Source: CAD feature listing. Evaluate the final solid. Frame: model axes, mm. A direction names the side the tool comes from. Give positions to 0.01 mm unless a question says otherwise; leave off trailing zeros. Order: outer loops, then holes, each group sorted by start corner. A loop starts at its lowest first (then second) coordinate and runs counter-clockwise, first axis right, second up. Notation, with made-up numbers: M 31,85.25 L 85,85.25 A12 ccw 85,108.25 Z; hole C 31.5,47 d1. An arc over 180 degrees is marked long. Answer in a Markdown table with one row per item. Add a question column.
(1) Mould query, pull axis X, two halves, no side actions, for faces 1 (the face through (3.45, -4.93, 0.74)), 2 (the face through (20, -23, 1.5)), 3 (the face through (40, -49, 2)). Classes: pulls with the +X half, pulls with the -X half, needs draft (parallel to the pull), parting line crosses it, or undercut.
(2) Material intervals for line 1 along Y through (x, z) = (5, 0.3); line 2 along Y through (x, z) = (35, 2); line 3 along Z through (x, y) = (13, -20.5), sorted ascending.
(3) Section query B-B, the plane z = 3.5. Return loops of the section in (x, y).
(4) Section query C-C, the plane y = -12. Return loops of the section in (x, z), plus the area to 3 significant figures.
(5) Set-up query: faces 4 (the face through (20, -46, 4)), 5 (the face through (36.478, -4.534, 0.74)). Return all of +Z, -Z, +X, -X, +Y, -Y with unobstructed straight access to the full face (end or side cutting, diameter ignored); none if empty.
(6) Pin query (flat end, axial travel): P1, Ø3.5, axis at x = 35, y = -35, coming from the +Z side; P2, Ø3, axis at x = 5, y = -35, coming from the +Z side; P3, Ø1.5, axis at x = 16.5, z = 5, coming from the +Y side. Return the tip coordinate at first contact, or that it passes through.
(7) Section query A-A, the plane y = -35. Return loops of the section in (x, z), plus the area to 3 significant figures.
from build123d import *

# Parameters (mm, degrees)
SKETCH_1_W          = 40
SKETCH_1_H          = 70
SKETCH_1_R          = 1.55
EXTRUDE_1_DEPTH     = 1.5
SKETCH_2_W          = 40
SKETCH_2_H          = 24
EXTRUDE_2_DEPTH     = 5
SKETCH_3_R          = 1.55
CUT_EXTRUDE_1_DEPTH = 25
FILLET_1_R          = 5


with BuildPart() as part:
    # 草图1 → 凸台-拉伸1 (new body)
    with BuildSketch(Plane.XY):
        with Locations((20, -35)):
            Rectangle(SKETCH_1_W, SKETCH_1_H)
        with Locations((5, -5)):
            Circle(SKETCH_1_R, mode=Mode.SUBTRACT)
        with Locations((35, -5)):
            Circle(SKETCH_1_R, mode=Mode.SUBTRACT)
        with Locations((5, -35)):
            Circle(SKETCH_1_R, mode=Mode.SUBTRACT)
        with Locations((35, -35)):
            Circle(SKETCH_1_R, mode=Mode.SUBTRACT)
        with Locations((5, -65)):
            Circle(SKETCH_1_R, mode=Mode.SUBTRACT)
        with Locations((35, -65)):
            Circle(SKETCH_1_R, mode=Mode.SUBTRACT)
    extrude(amount=EXTRUDE_1_DEPTH)

    # 草图2 → 凸台-拉伸2 (add)
    with BuildSketch(Plane.XY.offset(1.5)):
        with Locations((20, -58)):
            Rectangle(SKETCH_2_W, SKETCH_2_H)
    extrude(amount=EXTRUDE_2_DEPTH)

    # 草图3 → 切除-拉伸1 (cut)
    with BuildSketch(Plane(origin=(0, 0, 1.5), x_dir=(-1, 0, 0), z_dir=(0, 0, -1))):
        with Locations(Location((-35, -65, 0), (0, 0, 180))):
            Circle(SKETCH_3_R)
        with Locations(Location((-5, -65, 0), (0, 0, 180))):
            Circle(SKETCH_3_R)
    extrude(amount=-CUT_EXTRUDE_1_DEPTH, mode=Mode.SUBTRACT)

    # 圆角1
    fillet_1_edges = [part.edges().sort_by_distance(p)[0] for p in [
        (0, 0, 0.75),
        (40, 0, 0.75),
        (40, -70, 3.25),
        (0, -70, 3.25),
    ]]
    fillet(fillet_1_edges, radius=FILLET_1_R)


solid = part.part
Values follow:
| question | item | result |
|---|---|---|
| 1 | face 1 | undercut |
| 1 | face 2 | needs draft |
| 1 | face 3 | pulls with the +X half |
| 2 | line 1 | y = -70 to -66.55, -63.45 to -36.55, -33.45 to -6.55, -3.45 to 0 |
| 2 | line 2 | y = -70 to -66.55, -63.45 to -46 |
| 2 | line 3 | z = 0 to 1.5 |
| 3 | outline | M 0,-65 A5 ccw 5,-70 L 35,-70 A5 ccw 40,-65 L 40,-46 L 0,-46 Z; hole C 5,-65 d3.1; hole C 35,-65 d3.1 |
| 4 | outline | M 0,0 L 40,0 L 40,1.5 L 0,1.5 Z |
| 4 | area | 60.0 mm² |
| 5 | face 4 | +Z, +X, -X, +Y |
| 5 | face 5 | +Z, -Z |
| 6 | P1 | stops at z = 1.5 |
| 6 | P2 | passes through |
| 6 | P3 | stops at y = -46 |
| 7 | outline | M 0,0 L 3.45,0 L 3.45,1.5 L 0,1.5 Z; M 6.55,0 L 33.45,0 L 33.45,1.5 L 6.55,1.5 Z; M 36.55,0 L 40,0 L 40,1.5 L 36.55,1.5 Z |
| 7 | area | 50.7 mm² |
